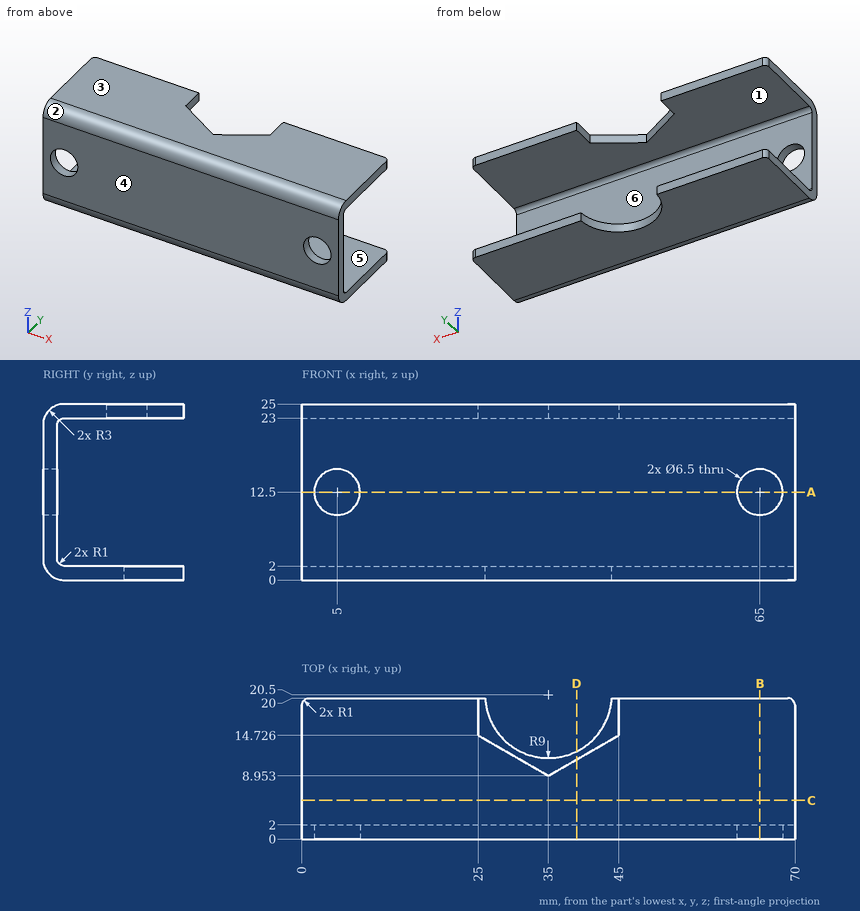
Drawing for the job (mm, zero at the part's lowest x, y, z). A direction names the side the tool comes from. Coordinates: 2 decimals unless noted, no trailing zeros. Order: outer loops, then holes, each group sorted by start corner. A loop starts at its lowest first (then second) coordinate and runs counter-clockwise, first axis right, second up.
Item 1: Band-saw the part on B-B on x = 65. List the corners of the cut face in (y, z).
Check sheet entries:
outline: (0, 3) arc R3 ccw to (3, 0) - (20, 0) - (20, 2) - (3, 2) arc R1 cw to (2, 3) - (2, 9.25) - (0, 9.25) - close; (0, 15.75) - (2, 15.75) - (2, 22) arc R1 cw to (3, 23) - (20, 23) - (20, 25) - (3, 25) arc R3 ccw to (0, 22) - close
Item 2: Band-saw the part on A-A on z = 12.5. List the corners of the cut face in (x, y).
Check sheet entries:
outline: (0, 0) - (1.75, 0) - (1.75, 2) - (0, 2) - close; (8.25, 0) - (61.75, 0) - (61.75, 2) - (8.25, 2) - close; (68.25, 0) - (70, 0) - (70, 2) - (68.25, 2) - close
Item 3: 3-axis set-ups, long thin cutter, end or side, ignore diameter. For the marked faces 1 and 2: which of +Z, -Z, +X, -X, +Y, -Y reach the whole face in a straight line?
Check sheet entries:
face 1: +X, -X, +Y
face 2: +Z, +X, -X, -Y
Item 4: Two-plate mould, pull along Z, no slides. Class the marked faces 3, 4, 5 and 6: +Z half, -Z half, draft (parallel to the pull), parting line (faces both ways), or undercut.
Check sheet entries:
face 3: +Z half
face 4: draft
face 5: undercut
face 6: undercut
Item 5: Band-saw the part on C-C on y = 5.5. List the corners of the cut face in (x, z).
Check sheet entries:
outline: (0, 0) - (70, 0) - (70, 2) - (0, 2) - close; (0, 23) - (70, 23) - (70, 25) - (0, 25) - close
Item 6: Drill centre lines: L1, parallel to X at y = 1.3, z = 12.5; L2, parallel to Z at x = 17, y = 18.75; L3, parallel to Y at x = 37.5, z = 7.25. Where is each one in solid material? Low to high.
Check sheet entries:
L1: x = 0 to 1.75, 8.25 to 61.75, 68.25 to 70
L2: z = 0 to 2, 23 to 25
L3: y = 0 to 2
Item 7: Band-saw the part on D-D on x = 39. List the corners of the cut face in (y, z).
Check sheet entries:
outline: (0, 3) arc R3 ccw to (3, 0) - (12.44, 0) - (12.44, 2) - (3, 2) arc R1 cw to (2, 3) - (2, 22) arc R1 cw to (3, 23) - (11.26, 23) - (11.26, 25) - (3, 25) arc R3 ccw to (0, 22) - close
Item 8: Pin check, flat tip, straight feed: pin 1 Ø8.5 at (x, z) = (5, 12.5) entering from +Y. Stop position of the tip, or through.
Check sheet entries:
pin 1: stops at y = 2
